The drawing under review shows one solid part. Ordinate dimensions are in mm from its lowest x, y, z. A direction names the side the tool comes from. Coordinates: 2 decimals unless noted, no trailing zeros. Order: outer loops, then holes, each group sorted by start corner. A loop starts at its lowest first (then second) coordinate and runs counter-clockwise, first axis right, second up. Notation, with made-up numbers: (44, 65) -> (83, 65) arc R28 ccw to (83, 103) -> close; hole circle Ø6 at (-17.5, 89). An arc over 180 degrees is marked (long way). Use a Markdown table: item, result. Add a question column.
Q1. Add section A-A (x = 6). State the section outline as (y, z) points.
Q2. Add section B-B (z = 5.08). State the section outline as (x, y) points, then the cut area to 3 significant figures.
Q3. Machinability: for the marked faces 1 and 2, which of the approach directions +Z, -Z, +X, -X, +Y, -Y give a long, thin tool a straight path to every point of the face, cutting with its end or side? Answer none if there is none.
Q4. Wall thickness on probe 1 along Y at (x, z) = (0.7, 20.32); probe 2 along X at (y, z) = (1.3, 20.65); probe 3 along Z at (x, y) = (6, 1.5): over which ranges is each line inside the solid? List them lowest first.
Q5. Add section D-D (x = 10.25). State the section outline as (y, z) points.
Q6. Add section C-C (z = 22.5). State the section outline as (x, y) points.
Q7. Insertion check: pin 1 (3 mm diameter, centred on y = 9.525, z = 5.08, fed in from +X); pin 2 (8 mm diameter, centred on x = 10, z = 14.5, fed in from +Y). Each pin has a flat end and moves straight along its axis. Give the tip position at first contact, or say it passes through.
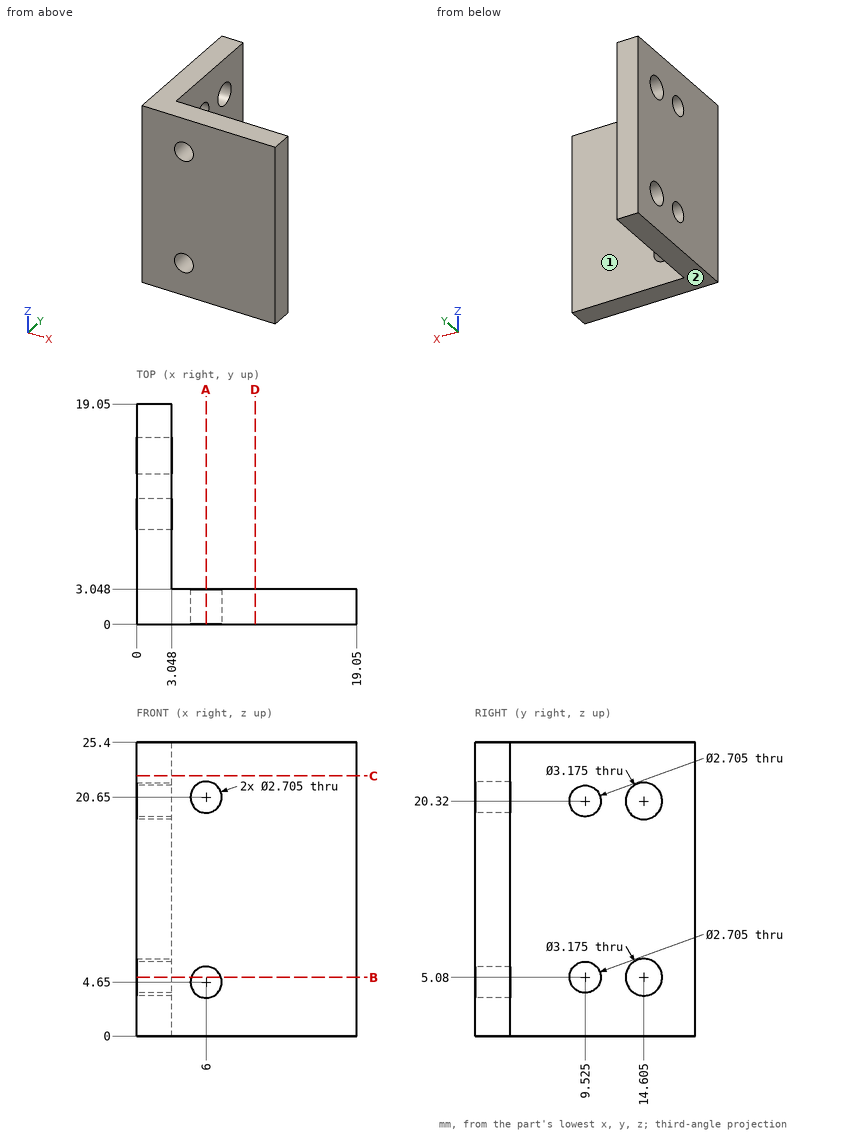
Established:
| question | item | result |
|---|---|---|
| 1 | outline | (0, 0) -> (3.05, 0) -> (3.05, 3.3) -> (0, 3.3) -> close; (0, 6) -> (3.05, 6) -> (3.05, 19.3) -> (0, 19.3) -> close; (0, 22) -> (3.05, 22) -> (3.05, 25.4) -> (0, 25.4) -> close |
| 2 | outline | (0, 0) -> (4.72, 0) -> (4.72, 3.05) -> (3.05, 3.05) -> (3.05, 8.17) -> (0, 8.17) -> close; (0, 10.88) -> (3.05, 10.88) -> (3.05, 13.02) -> (0, 13.02) -> close; (0, 16.19) -> (3.05, 16.19) -> (3.05, 19.05) -> (0, 19.05) -> close; (7.28, 0) -> (19.05, 0) -> (19.05, 3.05) -> (7.28, 3.05) -> close |
| 2 | area | 81.1 mm^2 |
| 3 | face 1 | +Z, -Z, +X, +Y |
| 3 | face 2 | -Z, +X, -X, +Y, -Y |
| 4 | probe 1 | 0 to 8.17, 10.88 to 13.02, 16.19 to 19.05 |
| 4 | probe 2 | 0 to 4.65, 7.35 to 19.05 |
| 4 | probe 3 | 0 to 3.3, 6 to 19.3, 22 to 25.4 |
| 5 | outline | (0, 0) -> (3.05, 0) -> (3.05, 25.4) -> (0, 25.4) -> close |
| 6 | outline | (0, 0) -> (19.05, 0) -> (19.05, 3.05) -> (3.05, 3.05) -> (3.05, 19.05) -> (0, 19.05) -> close |
| 7 | pin 1 | x = 3.05 |
| 7 | pin 2 | y = 3.05 |
